```python
from build123d import *

# Parameters (mm, degrees)
SKETCH1_R           = 1.75
SKETCH1_W           = 7.2
SKETCH1_H           = 5.4
BOSS_EXTRUDE1_DEPTH = 5
FILLET5_RADIUS      = 10
FILLET5_LENGTH      = 5
FILLET2_R           = 5.4
FILLET6_R           = 5.4
SKETCH3_W           = 35
SKETCH3_H           = 20
SKETCH3_W_2         = 23
SKETCH3_H_2         = 13
BOSS_EXTRUDE4_DEPTH = 5.5
SKETCH5_W           = 23
SKETCH5_H           = 13
CUT_EXTRUDE1_DEPTH  = 3.5
CUT_EXTRUDE2_DEPTH  = 76.201396264
SKETCH9_R           = 1
CUT_EXTRUDE4_DEPTH  = 7
SKETCH10_W          = 36
SKETCH10_H          = 5
CUT_EXTRUDE5_DEPTH  = 10
FILLET10_R          = 4
SKETCH11_W          = 44.4
SKETCH11_H          = 25
BOSS_EXTRUDE5_DEPTH = 5
SKETCH12_W          = 1.180339887
SKETCH12_H          = 5
BOSS_EXTRUDE6_DEPTH = 44.4
SKETCH13_R          = 0.75
CUT_EXTRUDE6_DEPTH  = 5


with BuildPart() as part:
    # Sketch1 → Boss-Extrude1 (new body)
    # profile 1 of 4: a face of its own
    with BuildSketch(Plane(origin=(0, 0, 0), x_dir=(1, 0, 0), z_dir=(0, 1, 0))):
        with BuildLine():
            Line((3.25, 25), (0, 25))
            Line((0, 25), (0, 15))
            Line((0, 15), (10, 0))
            Line((10, 0), (26, 0))
            Line((26, 0), (36, 15))
            Line((36, 15), (60, 15))
            Line((60, 15), (60, 25))
            Line((60, 25), (44.5, 25))
            Line((44.5, 25), (44.5, 19.6))
            Line((44.5, 19.6), (37.3, 19.6))
            Line((37.3, 19.6), (26.5, 19.6))
            Line((26.5, 19.6), (26.5, 25))
            Line((26.5, 25), (6.75, 25))
            ThreePointArc((6.75, 25), (5, 23.25), (3.25, 25))
        make_face()
        with Locations(Location((13, 5, 0), (0, 0, 270))):
            Circle(SKETCH1_R, mode=Mode.SUBTRACT)
        with Locations(Location((23, 5, 0), (0, 0, 270))):
            Circle(SKETCH1_R, mode=Mode.SUBTRACT)
    # profile 2 of 4: a face of its own
    with BuildSketch(Plane(origin=(0, 0, 0), x_dir=(1, 0, 0), z_dir=(0, 1, 0))):
        with BuildLine():
            Line((10, 45), (0, 33.819660113))
            Line((0, 33.819660113), (0, 25))
            Line((0, 25), (3.25, 25))
            ThreePointArc((3.25, 25), (5, 26.75), (6.75, 25))
            Line((6.75, 25), (26.5, 25))
            Line((26.5, 25), (26.5, 30.4))
            Line((26.5, 30.4), (37.3, 30.4))
            Line((37.3, 30.4), (44.5, 30.4))
            Line((44.5, 30.4), (44.5, 25))
            Line((44.5, 25), (60, 25))
            Line((60, 25), (60, 35))
            Line((60, 35), (36, 35))
            Line((36, 35), (26, 45))
            Line((26, 45), (10, 45))
        make_face()
    # profile 3 of 4: a face of its own
    with BuildSketch(Plane(origin=(0, 0, 0), x_dir=(1, 0, 0), z_dir=(0, 1, 0))):
        with Locations((40.9, 27.7)):
            Rectangle(SKETCH1_W, SKETCH1_H)
    # profile 4 of 4: a face of its own
    with BuildSketch(Plane(origin=(0, 0, 0), x_dir=(1, 0, 0), z_dir=(0, 1, 0))):
        with Locations((40.9, 22.3)):
            Rectangle(SKETCH1_W, SKETCH1_H)
    extrude(amount=BOSS_EXTRUDE1_DEPTH)

    # Fillet5: full round fillet: the end face becomes a half cylinder, R = half its width
    fillet5_face = Plane((60, 2.5, -25), x_dir=(0, -1, 0), z_dir=(1, 0, 0))  # on the end face: x along it, z out of the body
    fillet5_slab = fillet5_face.offset(-FILLET5_RADIUS / 2) * Box(FILLET5_LENGTH, 2 * FILLET5_RADIUS, FILLET5_RADIUS, mode=Mode.PRIVATE)  # the body's end, R deep
    fillet5_round = Plane((50, 2.5, -25), x_dir=(1, 0, 0), z_dir=(0, -1, 0)) * Cylinder(FILLET5_RADIUS, FILLET5_LENGTH, mode=Mode.PRIVATE)  # its axis R under the face
    add(fillet5_slab - fillet5_round, mode=Mode.SUBTRACT)

    # Fillet2
    fillet2_edges = [part.edges().sort_by_distance(p)[0] for p in [
        (26.5, 2.5, -30.4),
        (26.5, 2.5, -19.6),
    ]]
    fillet(fillet2_edges, radius=FILLET2_R - 0.0001)  # a hair under: the kernel refuses the full size

    # Fillet6
    fillet6_edges = [part.edges().sort_by_distance(p)[0] for p in [
        (37.3, 2.5, -19.6),
        (37.3, 2.5, -30.4),
    ]]
    fillet(fillet6_edges, radius=FILLET6_R - 0.0001)  # a hair under: the kernel refuses the full size

    # Sketch3 → Boss-Extrude4 (add)
    with BuildSketch(Plane.XZ):
        with Locations((26.9, -25)):
            Rectangle(SKETCH3_W, SKETCH3_H)
        with Locations((26.9, -25)):
            Rectangle(SKETCH3_W_2, SKETCH3_H_2, mode=Mode.SUBTRACT)
    extrude(amount=BOSS_EXTRUDE4_DEPTH)

    # Sketch5 → Cut-Extrude1 (cut)
    with BuildSketch(Plane.XZ):
        with Locations((26.9, -25)):
            Rectangle(SKETCH5_W, SKETCH5_H)
    extrude(amount=-CUT_EXTRUDE1_DEPTH, mode=Mode.SUBTRACT)

    # Sketch6 → Cut-Extrude2 (cut, through all)
    with BuildSketch(Plane.XZ):
        with BuildLine():
            Line((44.4, -15), (44.4, -35))
            Line((44.4, -35), (50, -35))
            ThreePointArc((50, -35), (60, -25), (50, -15))
            Line((50, -15), (44.4, -15))
        make_face()
    extrude(amount=-CUT_EXTRUDE2_DEPTH, mode=Mode.SUBTRACT)

    # Sketch9 → Cut-Extrude4 (cut)
    with BuildSketch(Plane.XZ.offset(5.5)):
        with Locations(Location((13.1, -25, 0), (0, 0, 270))):
            Circle(SKETCH9_R)
        with Locations(Location((40.7, -25, 0), (0, 0, 270))):
            Circle(SKETCH9_R)
    extrude(amount=-CUT_EXTRUDE4_DEPTH, mode=Mode.SUBTRACT)

    # Sketch10 → Cut-Extrude5 (cut)
    with BuildSketch(Plane(origin=(0, 0, -45), x_dir=(-1, 0, 0), z_dir=(0, 0, -1))):
        with Locations((-18, 2.5)):
            Rectangle(SKETCH10_W, SKETCH10_H)
    extrude(amount=-CUT_EXTRUDE5_DEPTH, mode=Mode.SUBTRACT)

    # Fillet10
    fillet10_edges = [part.edges().sort_by_distance(p)[0] for p in [
        (36, 2.5, -15),
        (26, 2.5, 0),
        (10, 2.5, 0),
        (0, 2.5, -15),
        (44.4, -0.25, -15),
        (9.4, -2.75, -15),
    ]]
    fillet(fillet10_edges, radius=FILLET10_R)

    # Sketch11 → Boss-Extrude5 (add)
    with BuildSketch(Plane(origin=(0, 0, -35), x_dir=(-1, 0, 0), z_dir=(0, 0, -1))):
        with Locations((-22.2, -7.5)):
            Rectangle(SKETCH11_W, SKETCH11_H)
    extrude(amount=BOSS_EXTRUDE5_DEPTH)

    # Sketch12 → Boss-Extrude6 (add)
    with BuildSketch(Plane.ZY):
        with Locations((-34.409830056, 2.5)):
            Rectangle(SKETCH12_W, SKETCH12_H)
    extrude(amount=-BOSS_EXTRUDE6_DEPTH)

    # Sketch13 → Cut-Extrude6 (cut)
    with BuildSketch(Plane(origin=(0, 0, -40), x_dir=(-1, 0, 0), z_dir=(0, 0, -1))):
        with Locations((-26, 0.5)):
            Circle(SKETCH13_R)
        with Locations((-10, 0.5)):
            Circle(SKETCH13_R)
        with Locations((-10, -15.5)):
            Circle(SKETCH13_R)
        with Locations((-26, -15.5)):
            Circle(SKETCH13_R)
    extrude(amount=-CUT_EXTRUDE6_DEPTH, mode=Mode.SUBTRACT)


solid = part.part
```
Source: CAD feature listing. Evaluate the final solid. Frame: model axes, mm. A direction names the side the tool comes from. Round coordinates to 2 decimals unless told otherwise and drop trailing zeros. Loops run counter-clockwise (first coordinate to the right, second up) from the corner with the lowest first, then second, coordinate; pieces in that order, holes last. Notation, with made-up numbers: M 44.5,72.25 L 69.5,72.25 A24 cw 69.5,86.25 Z; hole C 11.5,-38 d5. An arc over 180 degrees is marked long. Use a Markdown table: item, result. Add a question column.
1. Line query: line 1 (Y direction, x = 10, z = -38.4); line 2 (X direction, y = 2.1, z = -5); line 3 (X direction, y = -3.5, z = -25). Output: solid intervals per line, ascending.
2. Reachability of faces 1 (the cylindrical face through (28.04, 4.26, -28.776)), 2 (the flat face through (15, 0, -14)), 3 (the flat face through (18, 2, 0)), 4 (the cylindrical face through (26.595, 0.044, -37.535)), 5 (the flat face through (41, 1.5, -25)) from +Z, -Z, +X, -X, +Y, -Y: full face, straight path, thin tool, end or side. Return the list, or none.
3. Section query C-C on x = 23. Return the cut outline in (y, z), then the cut area to 4 significant figures.
4. Section query B-B on z = -5. Return the cut outline in (x, y).
5. Section query D-D on z = -22. Return the cut outline in (x, y).
6. Mould query, pull axis Z, two halves, no side actions, for faces 6 (the flat face through (0, -2, -36)), 7 (the flat face through (26, 1, -35)), 8 (the cylindrical face through (25.771, 2.535, -0.486)), 9 (the cylindrical face through (14.735, 2.465, -5.228)). Classes: pulls with the +Z half, pulls with the -Z half, needs draft (parallel to the pull), parting line crosses it, or undercut.
7. Contact query for flat-ended pins moving along their axis: P1, Ø2, axis at x = 26, y = 0.5, coming from the +Z side; P2, Ø6, axis at x = 9.5, y = -15.5, coming from the +Z side; P3, Ø1.5, axis at x = 37.5, z = -28.5, coming from the -Y side. Output: stop coordinate, or through.
8. Section query A-A on x = 5. Return the cut outline in (y, z), then the cut area to 3 significant figures.
Reported:
| question | item | result |
|---|---|---|
| 1 | line 1 | y = -20 to -16.25, -14.75 to -0.25, 1.25 to 5 |
| 1 | line 2 | x = 6.67 to 11.25, 14.75 to 21.25, 24.75 to 29.33 |
| 1 | line 3 | x = 9.4 to 12.1, 14.1 to 15.4, 38.4 to 39.7, 41.7 to 44.4 |
| 2 | face 1 | +Y, -Y |
| 2 | face 2 | +Z, -X, -Y |
| 2 | face 3 | +Z, +X, -X, +Y, -Y |
| 2 | face 4 | -Z |
| 2 | face 5 | -Y |
| 3 | outline | M -20,-40 L 5,-40 L 5,-6.75 L 0,-6.75 L 0,-15 L -5.5,-15 L -5.5,-18.5 L 3.5,-18.5 L 3.5,-31.5 L -5.5,-31.5 L -5.5,-35 L -20,-35 Z; M 0,-3.25 L 5,-3.25 L 5,0 L 0,0 Z |
| 3 | area | 275.5 mm² |
| 4 | outline | M 6.67,0 L 11.25,0 L 11.25,5 L 6.67,5 Z; M 14.75,0 L 21.25,0 L 21.25,5 L 14.75,5 Z; M 24.75,0 L 29.33,0 L 29.33,5 L 24.75,5 Z |
| 5 | outline | M 0,0 L 9.4,0 L 9.4,-5.5 L 15.4,-5.5 L 15.4,3.5 L 27.41,3.5 L 27.41,5 L 0,5 Z; M 36.39,3.5 L 38.4,3.5 L 38.4,-5.5 L 44.4,-5.5 L 44.4,5 L 36.39,5 Z |
| 6 | face 6 | needs draft |
| 6 | face 7 | pulls with the -Z half |
| 6 | face 8 | pulls with the +Z half |
| 6 | face 9 | undercut |
| 7 | P1 | stops at z = -0.17 |
| 7 | P2 | stops at z = -35 |
| 7 | P3 | stops at y = 3.5 |
| 8 | outline | M -20,-40 L 5,-40 L 5,-26.75 L 0,-26.75 L 0,-35 L -20,-35 Z; M 0,-23.25 L 5,-23.25 L 5,-7.5 L 0,-7.5 Z |
| 8 | area | 245 mm² |
